Work out the finished part from the listing and answer in its coordinate system (mm). Round coordinates to 2 decimals unless told otherwise and drop trailing zeros. Loops run counter-clockwise (first coordinate to the right, second up) from the corner with the lowest first, then second, coordinate; pieces in that order, holes last. Notation, with made-up numbers: (12.5, -5) - (64.5, -5) arc R31 ccw to (64.5, 20) - close; hole circle Ø10 at (-35, 19.5). An arc over 180 degrees is marked (long way). Use CSV: the item, a comma, the result in double quotes. Start each with the question number.
from build123d import *

# Parameters (mm, degrees)
SKETCH3_R                     = 19.304
SKETCH3_R_2                   = 2.55
BOSS_EXTRUDE1_DEPTH           = 6.35
TAP_DRILL_FOR_3_56_TAP1_D     = 2.0828
TAP_DRILL_FOR_3_56_TAP1_DEPTH = 7.62
TAP_DRILL_FOR_3_56_TAP1_TIP   = 0.625736249
TAP_DRILL_FOR_8_32_TAP2_D     = 3.4544


with BuildPart() as part:
    # Sketch3 → Boss-Extrude1 (new body)
    with BuildSketch(Plane.XY):
        with BuildLine():
            Line((-33.28, 35.82), (76.46, 35.82))
            ThreePointArc((76.46, 35.82), (78.256051224, 35.076051224), (79, 33.28))
            Line((79, 33.28), (79, -33.28))
            ThreePointArc((79, -33.28), (78.256051224, -35.076051224), (76.46, -35.82))
            Line((76.46, -35.82), (-33.28, -35.82))
            ThreePointArc((-33.28, -35.82), (-35.076051224, -35.076051224), (-35.82, -33.28))
            Line((-35.82, -33.28), (-35.82, 33.28))
            ThreePointArc((-35.82, 33.28), (-35.076051224, 35.076051224), (-33.28, 35.82))
        make_face()
        Circle(SKETCH3_R, mode=Mode.SUBTRACT)
        with Locations((23.57, 23.57)):
            Circle(SKETCH3_R_2, mode=Mode.SUBTRACT)
        with Locations((-23.57, 23.57)):
            Circle(SKETCH3_R_2, mode=Mode.SUBTRACT)
        with Locations((-23.57, -23.57)):
            Circle(SKETCH3_R_2, mode=Mode.SUBTRACT)
        with Locations((23.57, -23.57)):
            Circle(SKETCH3_R_2, mode=Mode.SUBTRACT)
    extrude(amount=BOSS_EXTRUDE1_DEPTH)

    # Tap Drill for #3-56 Tap1
    with Locations(Plane(origin=(0, 0, 6.35), x_dir=(-1, 0, 0), z_dir=(0, 0, 1))):
        with Locations((-30.8029, 4.82), (-34.544, -32.645), (-16.764, -32.645), (-30.8029, -25.66)):
            Hole(TAP_DRILL_FOR_3_56_TAP1_D / 2, depth=TAP_DRILL_FOR_3_56_TAP1_DEPTH)
            with Locations((0, 0, -(TAP_DRILL_FOR_3_56_TAP1_DEPTH + TAP_DRILL_FOR_3_56_TAP1_TIP / 2))):  # 118° drill point
                Cone(0, TAP_DRILL_FOR_3_56_TAP1_D / 2, TAP_DRILL_FOR_3_56_TAP1_TIP, mode=Mode.SUBTRACT)

    # Tap Drill for #8-32 Tap2 (through all)
    with Locations(Plane(origin=(0, 0, 0), x_dir=(-1, 0, 0), z_dir=(0, 0, -1))):
        with Locations((-44.202, 23.12), (-44.202, -23.12)):
            Hole(TAP_DRILL_FOR_8_32_TAP2_D / 2)


solid = part.part
Item 1: The mould has two halves that part along X. Classify faces 1 (the cylindrical face through (78.236, 35.096, 3.131)), 2 (the cylindrical face through (-21.214, 22.593, 3.131)), 3 (the cylindrical face through (-35.096, 35.056, 3.131)), 4 (the cylindrical face through (-21.214, -24.547, 3.131)): pulls with the +X half, pulls with the -X half, needs draft (parallel to the pull), parting line crosses it, or undercut.
Item 2: A cutting plane is placed at C-C (z = 1.5). State how many separate pieces and enclosed holes the cut face has, plus the area to 3 significant figures.
Item 3: A cutting plane is placed at A-A (y = 0). Determine the outline of the cut face in (x, z), plus the area to 3 significant figures.
Item 4: Find the intervals of material crossed by probe 1 along Y at (x, z) = (-23.57, 3); probe 2 along X at (y, z) = (24.5, 4); probe 3 along X at (y, z) = (25.66, 3.25), in increasing order. Write a range as [from, to].
Item 5: A cutting plane is placed at B-B (x = 23.57). Determine the outline of the cut face in (y, z).
Item 6: A cutting plane is placed at D-D (x = 1.5). Determine the outline of the cut face in (y, z).
Result sheet:
1,face 1,"pulls with the +X half"
1,face 2,"undercut"
1,face 3,"pulls with the -X half"
1,face 4,"undercut"
2,separate pieces,"1"
2,enclosed holes,"11"
2,area,"6,940 mm^2"
3,outline,"(-35.82, 0) - (-19.3, 0) - (-19.3, 6.35) - (-35.82, 6.35) - close; (19.3, 0) - (79, 0) - (79, 6.35) - (19.3, 6.35) - close"
3,area,"484 mm^2"
4,probe 1,"[-35.82, -26.12], [-21.02, 21.02], [26.12, 35.82]"
4,probe 2,"[-35.82, -25.94], [-21.2, 21.2], [25.94, 43.16], [45.24, 79]"
4,probe 3,"[-35.82, -25.03], [-22.11, 22.11], [25.03, 29.76], [31.84, 79]"
5,outline,"(-35.82, 0) - (-26.12, 0) - (-26.12, 6.35) - (-35.82, 6.35) - close; (-21.02, 0) - (21.02, 0) - (21.02, 6.35) - (-21.02, 6.35) - close; (26.12, 0) - (35.82, 0) - (35.82, 6.35) - (26.12, 6.35) - close"
6,outline,"(-35.82, 0) - (-19.25, 0) - (-19.25, 6.35) - (-35.82, 6.35) - close; (19.25, 0) - (35.82, 0) - (35.82, 6.35) - (19.25, 6.35) - close"
